Check sheet for the modelled part. Datum: model origin and axes. Units: mm. Face numbers are marked on the shaded views. A direction names the side the tool comes from. Round coordinates to 2 decimals unless told otherwise and drop trailing zeros. Write each loop counter-clockwise with the first axis right and the second up, starting at its lowest first coordinate (ties: lowest second). Pieces come first, ordered by that corner, then holes. Notation, with made-up numbers: (19, 72) - (26, 72) arc R27 cw to (26, 96) - close; hole circle Ø8 at (27, 49). An arc over 180 degrees is marked (long way). Answer as a JSON object with one key per item and string values. Group by question number.
Item 1: Gauge pin test, flat end, axial feed: P1, Ø8, axis at x = -52, z = -7.5, coming from the -Y side. Record the tip position at first contact, or that the pin passes through.
Item 2: Sectioned sample at B-B on x = 32.5. Record the boundary of the cut face in (y, z).
Item 3: Sectioned sample at A-A on y = 62. Record the boundary of the cut face in (x, z).
Item 4: Thickness scan on line 1 (Z direction, x = -45, y = 6); line 2 (X direction, y = 76.5, z = -15); line 3 (Y direction, x = 37, z = -10). Record the ranges inside material, lowest first.
Item 5: Release check for a two-part mould opening along Z. For the marked faces 1, 2, 3 and 4 record: pulls with the +Z half, pulls with the -Z half, needs draft (parallel to the pull), parting line crosses it, or undercut.
Item 6: Set-up check for the marked faces 5 and 6: record each of +Z, -Z, +X, -X, +Y, -Y from which the full face is reachable in a straight line by a thin tool's end or side.
Item 7: Sectioned sample at C-C on z = 10. Record the boundary of the cut face in (x, y), plus the area to 3 significant figures.
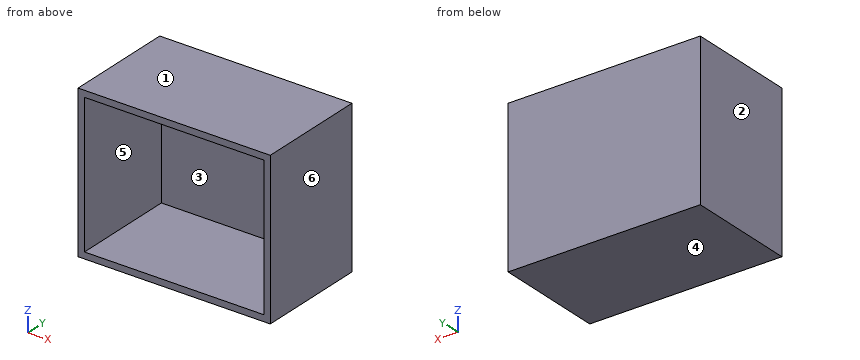
Autodesk Inventor part; units mm, degrees
ref_plane "YZ Plane" through (0, 0, 0) normal (1, 0, 0) x (0, 1, 0)
ref_plane "XZ Plane" through (0, 0, 0) normal (0, 1, 0) x (-1, 0, 0)
ref_plane "XY Plane" through (0, 0, 0) normal (0, 0, 1) x (1, 0, 0)
sketch "Sketch1" plane through (0, 0, 0) normal (0, 1, 0) x (-1, 0, 0)
  line L0 (-75, 60) -> (75, 60)
  line L1 (75, 60) -> (75, -60)
  line L2 (75, -60) -> (-75, -60)
  line L3 (-75, -60) -> (-75, 60)
  line L4 (-75, 60) -> (75, -60) construction
  line L5 (75, 60) -> (-75, -60) construction
  line L6 (-70, 55) -> (70, 55)
  line L7 (70, 55) -> (70, -55)
  line L8 (70, -55) -> (-70, -55)
  line L9 (-70, -55) -> (-70, 55)
  line L10 (-70, 55) -> (70, -55) construction
  line L11 (70, 55) -> (-70, -55) construction
  point P0 (0, 0)
  dimension "d0" = 150
  dimension "d1" = 120
  dimension "d2" = 140
  dimension "d3" = 110
  dimension "d8" = 5
extrude "Extrusion1" add sketch "Sketch1" along normal blind 86 contours L0 L1 L2 L3 | L6 L7 L8 L9
extrude "Extrusion2" cut sketch "Sketch1" along normal blind 81 contours L6 L7 L8 L9
properties part number "Stand of Shooting"
Completed:
{
 "1": {"P1": "y = 81"},
 "2": {"outline": "(0, -60) - (86, -60) - (86, 60) - (0, 60) - (0, 55) - (81, 55) - (81, -55) - (0, -55) - close"},
 "3": {"outline": "(-75, -60) - (75, -60) - (75, 60) - (-75, 60) - close; hole (-70, -55) - (70, -55) - (70, 55) - (-70, 55) - close"},
 "4": {"line 1": "-60 to -55, 55 to 60", "line 2": "-75 to -70, 70 to 75", "line 3": "81 to 86"},
 "5": {"face 1": "pulls with the +Z half", "face 2": "needs draft", "face 3": "undercut", "face 4": "pulls with the -Z half"},
 "6": {"face 5": "-Y", "face 6": "+Z, -Z, +X, +Y, -Y"},
 "7": {"outline": "(-75, 0) - (-70, 0) - (-70, 81) - (70, 81) - (70, 0) - (75, 0) - (75, 86) - (-75, 86) - close", "area": "1,560 mm²"}
}
